Geometry: final body of the model. Coordinates: model frame, mm. A direction names the side the tool comes from. Coordinates: 2 decimals unless noted, no trailing zeros. Loops run counter-clockwise (first coordinate to the right, second up) from the corner with the lowest first, then second, coordinate; pieces in that order, holes last. Notation, with made-up numbers: (24, 10) -> (83, 10) arc R24 cw to (83, 43) -> close; hole circle Ø8 at (-1, -16). An arc over 180 degrees is marked (long way). One line per item, written item: value. Start each with the question number.
Item 1: Ray query, probe 1 along X at (y, z) = (0, 5); probe 2 along X at (y, z) = (-12, -17); probe 3 along X at (y, z) = (-9.5, 82). Return the intervals inside material, ascending. Write a range as from..to.
Item 2: Mould query, pull axis X, two halves, no side actions, for faces 6 (the flat face through (-3, 1.308, 1)), 7 (the cylindrical face through (-35.134, -18.496, 1.4)). Classes: +X half, -X half, draft (parallel to the pull), parting line (faces both ways), or undercut.
Item 3: Set-up query: faces 1 (the flat face through (53, -1.692, 1)), 2 (the flat face through (-4, -1, 100)), 3 (the flat face through (-60, -1.692, 1)), 4 (the flat face through (52, 1.308, 1)), 5 (the flat face through (-3, -1.692, 1)). Return all of +Z, -Z, +X, -X, +Y, -Y with unobstructed straight access to the full face (end or side cutting, diameter ignored); none if empty.
Item 4: Section query C-C on x = 51. Return loops of the section in (y, z), then the cut area to 3 significant figures.
Item 5: Section query D-D on x = -25. Return loops of the section in (y, z).
Item 6: Section query B-B on z = -23. Return loops of the section in (x, y), then the cut area to 3 significant figures.
Item 7: Contact query for flat-ended pins moving along their axis: pin 1 Ø10 at (x, y) = (-35, -6.5) entering from +Z; pin 2 Ø10.5 at (x, z) = (-61.5, 0.5) entering from -Y; pin 3 Ø10 at (y, z) = (-8, 18) entering from +X; pin 4 Ø5 at (x, z) = (-27, 50.5) entering from +Y. Output: stop coordinate, or through.
Item 8: Section query A-A on y = -11.25. Return loops of the section in (x, z).
from build123d import *

# Parameters (mm, degrees)
F1_DEPTH      = 100
F1_DEPTH_BACK = 100


with BuildPart() as f1:
    # F0 (on Top) → F1 (new body, two sides)
    with BuildSketch(Plane.XY) as f1_sk:
        with BuildLine():
            ThreePointArc((-18.302896, 1.308424), (-34.750936, -16.5), (-51.198977, 1.308424))
            Line((-51.198977, 1.308424), (-53.204609, 1.308424))
            Line((-53.204609, 1.308424), (-66.198977, 1.308424))
            Line((-66.198977, 1.308424), (-66.198977, -1.691576))
            Line((-66.198977, -1.691576), (-53.173438, -1.691576))
            ThreePointArc((-53.173438, -1.691576), (-34.750936, -18.5), (-16.328435, -1.691576))
            Line((-16.328435, -1.691576), (9.722642, -1.691576))
            ThreePointArc((9.722642, -1.691576), (28.145144, -18.5), (46.567646, -1.691576))
            Line((46.567646, -1.691576), (59.593184, -1.691576))
            Line((59.593184, -1.691576), (59.593184, 1.308424))
            Line((59.593184, 1.308424), (46.598816, 1.308424))
            Line((46.598816, 1.308424), (44.593184, 1.308424))
            ThreePointArc((44.593184, 1.308424), (28.145144, -16.5), (11.697104, 1.308424))
            Line((11.697104, 1.308424), (9.691472, 1.308424))
            Line((9.691472, 1.308424), (-16.297264, 1.308424))
            Line((-16.297264, 1.308424), (-18.302896, 1.308424))
        make_face()
    extrude(amount=F1_DEPTH)
    extrude(f1_sk.sketch, amount=-F1_DEPTH_BACK)


solid = f1.part
Reply:
1. probe 1: x = -66.2..-51.25, -18.25..11.65, 44.65..59.59
1. probe 2: x = -48.83..-46.08, -23.43..-20.67, 14.07..16.82, 39.47..42.23
1. probe 3: x = -50.63..-48.24, -21.26..-18.88, 12.27..14.65, 41.64..44.02
2. face 6: draft
2. face 7: undercut
3. face 1: +Z, -Z, +X, -Y
3. face 2: +Z, +X, -X, +Y, -Y
3. face 3: +Z, -Z, -X, -Y
3. face 4: +Z, -Z, +X, -X, +Y
3. face 5: +Z, -Z, -Y
4. outline: (-1.69, -100) -> (1.31, -100) -> (1.31, 100) -> (-1.69, 100) -> close
4. area: 600 mm²
5. outline: (-15.72, -100) -> (-13.31, -100) -> (-13.31, 100) -> (-15.72, 100) -> close
6. outline: (-66.2, -1.69) -> (-53.17, -1.69) arc R18.5 ccw to (-16.33, -1.69) -> (9.72, -1.69) arc R18.5 ccw to (46.57, -1.69) -> (59.59, -1.69) -> (59.59, 1.31) -> (44.59, 1.31) arc R16.5 cw (long way) to (11.7, 1.31) -> (-18.3, 1.31) arc R16.5 cw (long way) to (-51.2, 1.31) -> (-66.2, 1.31) -> close
6. area: 386 mm²
7. pin 1: passes through
7. pin 2: stops at y = -1.69
7. pin 3: stops at x = 46.4
7. pin 4: stops at y = -12.93
8. outline: (-49.44, -100) -> (-46.82, -100) -> (-46.82, 100) -> (-49.44, 100) -> close; (-22.68, -100) -> (-20.06, -100) -> (-20.06, 100) -> (-22.68, 100) -> close; (13.46, -100) -> (16.08, -100) -> (16.08, 100) -> (13.46, 100) -> close; (40.22, -100) -> (42.83, -100) -> (42.83, 100) -> (40.22, 100) -> close
